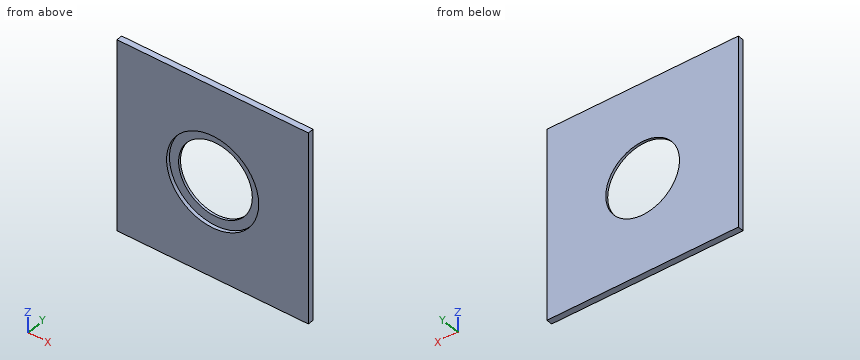
```python
from build123d import *

# Parameters (mm, degrees)
F0_W     = 101.6
F0_H     = 101.6
F1_DEPTH = 3.175
F2_R     = 19.558
F3_DEPTH = 3.176
F4_R     = 24.4475
F5_DEPTH = 1.905


with BuildPart() as f1:
    # F0 (on Front) → F1 (new body)
    with BuildSketch(Plane.XZ):
        Rectangle(F0_W, F0_H)
    extrude(amount=F1_DEPTH)

    # F2 (on face) → F3 (cut, through all)
    with BuildSketch(Plane.XZ.offset(3.175)):
        Circle(F2_R)
    extrude(amount=-F3_DEPTH, mode=Mode.SUBTRACT)

    # F4 (on face) → F5 (cut)
    with BuildSketch(Plane.XZ.offset(3.175)):
        Circle(F4_R)
    extrude(amount=-F5_DEPTH, mode=Mode.SUBTRACT)


solid = f1.part
```
Geometry: final body of the model. Coordinates: model frame, mm. Coordinates: 2 decimals unless noted, no trailing zeros. Order: outer loops, then holes, each group sorted by start corner. A loop starts at its lowest first (then second) coordinate and runs counter-clockwise, first axis right, second up. Notation, with made-up numbers: (73, 28.25) - (128, 28.25) arc R15 ccw to (128, 35.25) - close; hole circle Ø6 at (50, 48.25). An arc over 180 degrees is marked (long way). Return JSON: item names as keys, results as strings. Group by question number.
1. Cut plane B-B (z = 0). Output: boundary loops of the cut face in (x, y) (1 decimal).
2. Pin query (flat end, axial travel): pin 1 (10 mm diameter, centred on x = 4, z = -18.5, fed in from -Y). Return the tip coordinate at first contact, or that it passes through.
3. Cut plane C-C (y = -0.75). Output: boundary loops of the cut face in (x, z), plus the area to 3 significant figures.
4. Cut plane A-A (x = 0). Output: boundary loops of the cut face in (y, z) (1 decimal), plus the area to 3 significant figures.
5. Material intervals for line 1 along Z through (x, y) = (0, -0.95); line 2 along Z through (x, y) = (0, -2.35); line 3 along X through (y, z) = (-2.9, -21), sorted ascending. Write a range as [from, to].
Resolved:
{
 "1": {"outline": "(-50.8, -3.2) - (-24.4, -3.2) - (-24.4, -1.3) - (-19.6, -1.3) - (-19.6, 0) - (-50.8, 0) - close; (19.6, -1.3) - (24.4, -1.3) - (24.4, -3.2) - (50.8, -3.2) - (50.8, 0) - (19.6, 0) - close"},
 "2": {"pin 1": "stops at y = -1.27"},
 "3": {"outline": "(-50.8, -50.8) - (50.8, -50.8) - (50.8, 50.8) - (-50.8, 50.8) - close; hole circle Ø39.12 at (0, 0)", "area": "9,120 mm²"},
 "4": {"outline": "(-3.2, -50.8) - (0, -50.8) - (0, -19.6) - (-1.3, -19.6) - (-1.3, -24.4) - (-3.2, -24.4) - close; (-3.2, 24.4) - (-1.3, 24.4) - (-1.3, 19.6) - (0, 19.6) - (0, 50.8) - (-3.2, 50.8) - close", "area": "180 mm²"},
 "5": {"line 1": "z = [-50.8, -19.56], [19.56, 50.8]", "line 2": "z = [-50.8, -24.45], [24.45, 50.8]", "line 3": "x = [-50.8, -12.52], [12.52, 50.8]"}
}
